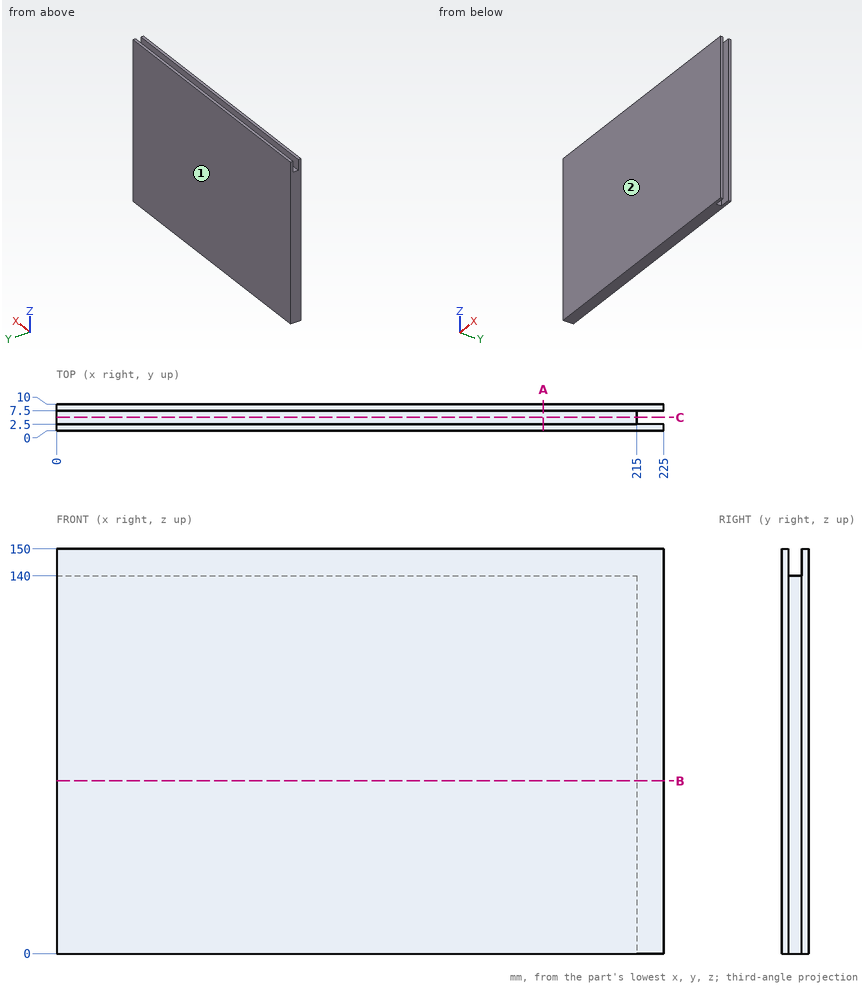
The figure shows three views and two pictorial views of one solid part (mm, origin at its lowest corner). Answer the questions. Round coordinates to 2 decimals unless told otherwise and drop trailing zeros. Loops run counter-clockwise (first coordinate to the right, second up) from the corner with the lowest first, then second, coordinate; pieces in that order, holes last. Notation, with made-up numbers: M -18,7.25 L -11,7.25 A16 cw -11,12.25 Z; hole C 73.25,84 d11. An arc over 180 degrees is marked long. Use CSV: the item, a comma, the result in double quotes.
Q1. Section C-C, the plane y = 5 is taken. Determine the outline of the cut face in (x, z), then the cut area to 3 significant figures.
Determined:
outline,"M 0,0 L 215,0 L 215,140 L 0,140 Z"
area,"30,100 mm2"
Q2. Each of these flat-tipped pins is pushed along its axis until it touches: pin 1 (2.5 mm diameter, centred on x = 122, y = 6, fed in from +Z); pin 2 (1.5 mm diameter, centred on y = 4.5, z = 99.5, fed in from +X); pin 3 (6 mm diameter, centred on x = 67, y = 7.5, fed in from -Z). Where does it stop, or does it pass through?
Determined:
pin 1,"z = 140"
pin 2,"x = 215"
pin 3,"z = 0"
Q3. Section A-A, the plane x = 180.5 is taken. Determine the outline of the cut face in (y, z), then the cut area to 3 significant figures.
Determined:
outline,"M 0,0 L 10,0 L 10,150 L 7.5,150 L 7.5,140 L 2.5,140 L 2.5,150 L 0,150 Z"
area,"1,450 mm2"
Q4. Section B-B, the plane z = 64 is taken. Determine the outline of the cut face in (x, y).
Determined:
outline,"M 0,0 L 225,0 L 225,2.5 L 215,2.5 L 215,7.5 L 225,7.5 L 225,10 L 0,10 Z"
Q5. Consider L1, parallel to Z at x = 151.5, y = 5.5; L2, parallel to X at y = 6, z = 64. Determine where each line is inside the solid, lowest interval first.
Determined:
L1,"0 to 140"
L2,"0 to 215"
Q6. The mould has two halves that part along Y. Classify the marked faces 1 and 2: pulls with the +Y half, pulls with the -Y half, needs draft (parallel to the pull), parting line crosses it, or undercut.
Determined:
face 1,"pulls with the +Y half"
face 2,"pulls with the -Y half"
